Verification items for this drawing (mm, ordinates from the low corner). A direction names the side the tool comes from. Round coordinates to 2 decimals unless told otherwise and drop trailing zeros. Write each loop counter-clockwise with the first axis right and the second up, starting at its lowest first coordinate (ties: lowest second). Pieces come first, ordered by that corner, then holes.
Item 1: Access from +Z, -Z, +X, -X, +Y, -Y to the whole of each face (thin tool, end or side, straight path). Record for the marked faces 1, 2 and 3.
Item 2: Cross-section at C-C (y = 25). Enter the section's corners in (x, z), then the cut area to 3 significant figures.
Item 3: Cross-section at B-B (x = 92). Enter the section's corners in (y, z), then the cut area to 3 significant figures.
Item 4: Depth check by flat-ended pin: P1, Ø2, axis at x = 47, z = 28.5, coming from the -Y side; P2, Ø12.5, axis at x = 95.25, z = 19.05, coming from the -Y side; P3, Ø3.5, axis at x = 3.5, y = 28.5, coming from the +Z side; P4, Ø6, axis at y = 21.5, z = 34, coming from the +X side. Enter the tip coordinate at first touch or a pass-through.
Item 5: Scan lines: probe 1 along X at (y, z) = (39, 19); probe 2 along Y at (x, z) = (37.5, 21); probe 3 along Z at (x, y) = (95.25, 37.75). Record each from-to range of solid material in increasing order.
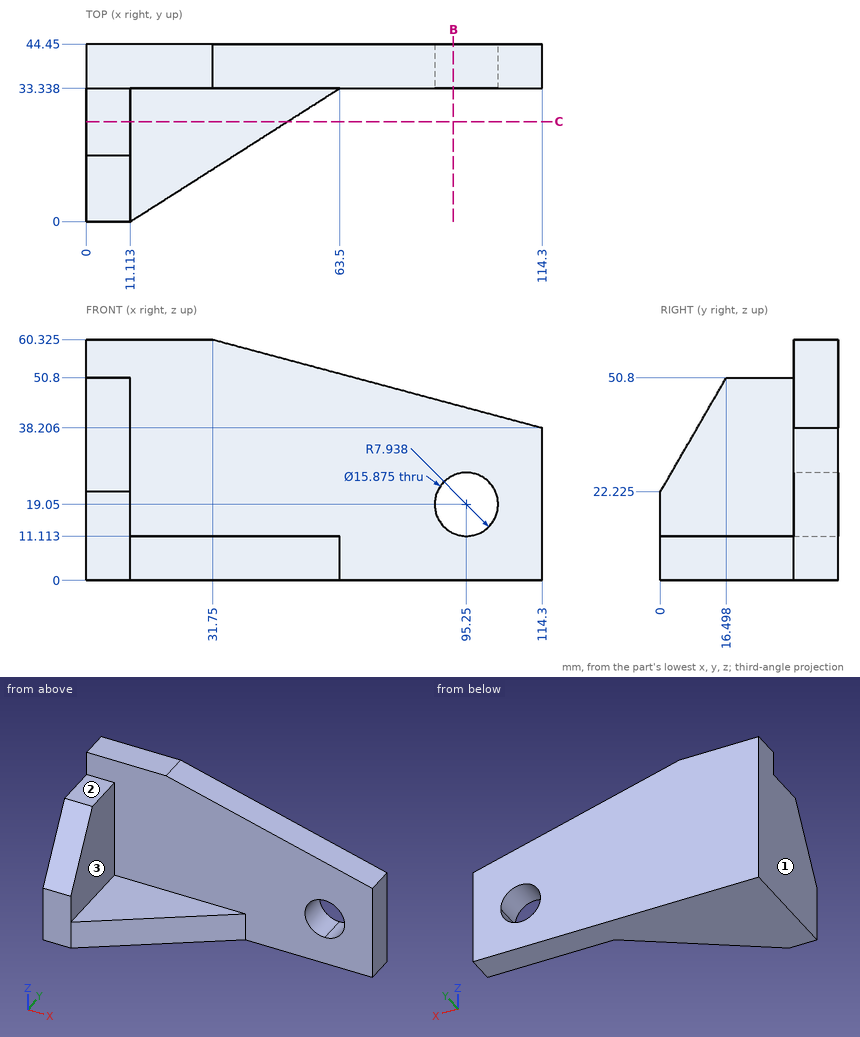
Resolved:
1. face 1: +Z, -Z, -X, +Y, -Y
1. face 2: +Z, +X, -X, -Y
1. face 3: +Z, +X, -Y
2. outline: (0, 0) - (50.4, 0) - (50.4, 11.11) - (11.11, 11.11) - (11.11, 50.8) - (0, 50.8) - close
2. area: 1,000 mm2
3. outline: (33.34, 0) - (44.45, 0) - (44.45, 11.81) - (33.34, 11.81) - close; (33.34, 26.29) - (44.45, 26.29) - (44.45, 44.18) - (33.34, 44.18) - close
3. area: 330 mm2
4. P1: stops at y = 33.34
4. P2: passes through
4. P3: stops at z = 50.8
4. P4: stops at x = 11.11
5. probe 1: x = 0 to 87.31, 103.19 to 114.3
5. probe 2: y = 33.34 to 44.45
5. probe 3: z = 0 to 11.11, 26.99 to 43.31
